```python
from build123d import *

# Parameters (mm, degrees)
SKETCH1_R           = 2.05
BOSS_EXTRUDE1_DEPTH = 4
FILLET1_R           = 1.4
CHAMFER1_SIZE       = 1.9
CUT_EXTRUDE1_DEPTH  = 1.8
SKETCH4_R           = 30
CUT_EXTRUDE2_DEPTH  = 87.446515392


with BuildPart() as part:
    # Sketch1 → Boss-Extrude1 (new body)
    with BuildSketch(Plane(origin=(0, 0, 0), x_dir=(1, 0, 0), z_dir=(0, 1, 0))):
        with BuildLine():
            Line((72.5, -41), (-72.5, -41))
            ThreePointArc((-72.5, -41), (-74.974873734, -39.974873734), (-76, -37.5))
            Line((-76, -37.5), (-76, 37.5))
            ThreePointArc((-76, 37.5), (-74.974873734, 39.974873734), (-72.5, 41))
            Line((-72.5, 41), (72.5, 41))
            ThreePointArc((72.5, 41), (74.974873734, 39.974873734), (76, 37.5))
            Line((76, 37.5), (76, -37.5))
            ThreePointArc((76, -37.5), (74.974873734, -39.974873734), (72.5, -41))
        make_face()
        with Locations(Location((-71.25, 36.2, 0), (0, 0, 270))):
            Circle(SKETCH1_R, mode=Mode.SUBTRACT)
        with Locations(Location((-71.25, -36.2, 0), (0, 0, 270))):
            Circle(SKETCH1_R, mode=Mode.SUBTRACT)
        with Locations(Location((71.25, -36.2, 0), (0, 0, 270))):
            Circle(SKETCH1_R, mode=Mode.SUBTRACT)
        with Locations(Location((71.25, 36.2, 0), (0, 0, 270))):
            Circle(SKETCH1_R, mode=Mode.SUBTRACT)
        with Locations(Location((0, 36.2, 0), (0, 0, 270))):
            Circle(SKETCH1_R, mode=Mode.SUBTRACT)
        with Locations(Location((0, -36.2, 0), (0, 0, 270))):
            Circle(SKETCH1_R, mode=Mode.SUBTRACT)
    extrude(amount=BOSS_EXTRUDE1_DEPTH)

    # Fillet1
    fillet1_edges = [part.edges().sort_by_distance(p)[0] for p in [
        (74.974873734, 4, 39.974873734),
        (76, 4, 0),
        (74.974873734, 4, -39.974873734),
        (0, 4, -41),
        (-74.974873734, 4, -39.974873734),
        (-76, 4, 0),
        (-74.974873734, 4, 39.974873734),
        (0, 4, 41),
    ]]
    fillet(fillet1_edges, radius=FILLET1_R)

    # Chamfer1
    # the kernel refuses this chamfer: 1.9 mm, written as the material it takes off along each edge
    with BuildSketch(Plane(origin=(71.25, 4, 36.2), x_dir=(0, 0, 1), z_dir=(-1, 0, 0))) as chamfer1_piece_1:
        Polygon((2.05 + CHAMFER1_SIZE, 0), (2.05, -CHAMFER1_SIZE), (2.05, 0), align=None)
    revolve(axis=Axis((71.25, 4, 36.2), (0, 1, 0)), mode=Mode.SUBTRACT)
    with BuildSketch(Plane(origin=(71.25, 4, -36.2), x_dir=(0, 0, 1), z_dir=(-1, 0, 0))) as chamfer1_piece_2:
        Polygon((2.05 + CHAMFER1_SIZE, 0), (2.05, -CHAMFER1_SIZE), (2.05, 0), align=None)
    revolve(axis=Axis((71.25, 4, -36.2), (0, 1, 0)), mode=Mode.SUBTRACT)
    with BuildSketch(Plane(origin=(-71.25, 4, 36.2), x_dir=(0, 0, 1), z_dir=(-1, 0, 0))) as chamfer1_piece_3:
        Polygon((2.05 + CHAMFER1_SIZE, 0), (2.05, -CHAMFER1_SIZE), (2.05, 0), align=None)
    revolve(axis=Axis((-71.25, 4, 36.2), (0, 1, 0)), mode=Mode.SUBTRACT)
    with BuildSketch(Plane(origin=(-71.25, 4, -36.2), x_dir=(0, 0, 1), z_dir=(-1, 0, 0))) as chamfer1_piece_4:
        Polygon((2.05 + CHAMFER1_SIZE, 0), (2.05, -CHAMFER1_SIZE), (2.05, 0), align=None)
    revolve(axis=Axis((-71.25, 4, -36.2), (0, 1, 0)), mode=Mode.SUBTRACT)
    with BuildSketch(Plane(origin=(0, 4, 36.2), x_dir=(0, 0, 1), z_dir=(-1, 0, 0))) as chamfer1_piece_5:
        Polygon((2.05 + CHAMFER1_SIZE, 0), (2.05, -CHAMFER1_SIZE), (2.05, 0), align=None)
    revolve(axis=Axis((0, 4, 36.2), (0, 1, 0)), mode=Mode.SUBTRACT)
    with BuildSketch(Plane(origin=(0, 4, -36.2), x_dir=(0, 0, 1), z_dir=(-1, 0, 0))) as chamfer1_piece_6:
        Polygon((2.05 + CHAMFER1_SIZE, 0), (2.05, -CHAMFER1_SIZE), (2.05, 0), align=None)
    revolve(axis=Axis((0, 4, -36.2), (0, 1, 0)), mode=Mode.SUBTRACT)

    # Sketch2 → Cut-Extrude1 (cut)
    with BuildSketch(Plane.XZ):
        with BuildLine():
            Line((-71.25, 33.35), (-72.5, 33.35))
            Line((-72.5, 33.35), (-72.5, -33.35))
            Line((-72.5, -33.35), (-71.25, -33.35))
            ThreePointArc((-71.25, -33.35), (-69.234745674, -34.184745674), (-68.4, -36.2))
            Line((-68.4, -36.2), (-68.4, -37.45))
            Line((-68.4, -37.45), (-2.85, -37.45))
            Line((-2.85, -37.45), (-2.85, -36.2))
            ThreePointArc((-2.85, -36.2), (0, -33.35), (2.85, -36.2))
            Line((2.85, -36.2), (2.85, -37.45))
            Line((2.85, -37.45), (68.4, -37.45))
            Line((68.4, -37.45), (68.4, -36.2))
            ThreePointArc((68.4, -36.2), (69.234745674, -34.184745674), (71.25, -33.35))
            Line((71.25, -33.35), (72.5, -33.35))
            Line((72.5, -33.35), (72.5, 33.35))
            Line((72.5, 33.35), (71.25, 33.35))
            ThreePointArc((71.25, 33.35), (69.234745674, 34.184745674), (68.4, 36.2))
            Line((68.4, 36.2), (68.4, 37.45))
            Line((68.4, 37.45), (2.85, 37.45))
            Line((2.85, 37.45), (2.85, 36.2))
            ThreePointArc((2.85, 36.2), (0, 33.35), (-2.85, 36.2))
            Line((-2.85, 36.2), (-2.85, 37.45))
            Line((-2.85, 37.45), (-68.4, 37.45))
            Line((-68.4, 37.45), (-68.4, 36.2))
            ThreePointArc((-68.4, 36.2), (-69.234745674, 34.184745674), (-71.25, 33.35))
        make_face()
    extrude(amount=-CUT_EXTRUDE1_DEPTH, mode=Mode.SUBTRACT)

    # Sketch4 → Cut-Extrude2 (cut, through all)
    with BuildSketch(Plane(origin=(0, 4, 0), x_dir=(1, 0, 0), z_dir=(0, 1, 0))):
        with Locations(Location((-35.625, 0, 0), (0, 0, 270))):
            Circle(SKETCH4_R)
        with Locations(Location((35.625, 0, 0), (0, 0, 270))):
            Circle(SKETCH4_R)
    extrude(amount=-CUT_EXTRUDE2_DEPTH, mode=Mode.SUBTRACT)


solid = part.part
```
CAD build for the part. Positions are in the model's coordinates, mm. A direction names the side the tool comes from. Round coordinates to 2 decimals unless told otherwise and drop trailing zeros. Write each loop counter-clockwise with the first axis right and the second up, starting at its lowest first coordinate (ties: lowest second). Pieces come first, ordered by that corner, then holes. Notation, with made-up numbers: (-21.5, 40.25) - (-14.5, 40.25) arc R31 cw to (-14.5, 68.25) - close; hole circle Ø1 at (-16.75, -18). An arc over 180 degrees is marked (long way). Write item = value, one per line. Start each with the question number.
Q1. Which spindle directions (+Z, -Z, +X, -X, +Y, -Y) get a long thin tool onto all of the face, cutting with end or side? Do faces 1 (the cylindrical face through (69.21, 0.89, -34.21)), 2 (the cylindrical face through (73.283, 1.035, 35.933)). Say none if no direction does.
Q2. Mould opens along X. For faces 3 (the flat face through (-1, 1, -41)), 4 (the cylindrical face through (-74.95, 1.28, 40)), 5 (the cylindrical face through (-70.634, 1.035, -34.245)) say: pulls with the +X half, pulls with the -X half, needs draft (parallel to the pull), parting line crosses it, or undercut.
Q3. Probe L1, parallel to X at y = 0.95, z = -36.2; L2, parallel to X at y = 2.4, z = 0 (3 decimals); L3, parallel to Z at x = 65, y = 1.45. List the from-to ranges inside material, lowest first. Write a range as from..to.
Q4. Band-saw the part on A-A (z = 0). Give the cut face in (x, y) (3 decimals), then the cut area to 3 significant figures.
Q5. Drop flat-ended pins along their axis: pin 1 (5.5 mm diameter, centred on x = 0, z = -36.2, fed in from +Y); pin 2 (3.5 mm diameter, centred on x = -71.25, z = -36.2, fed in from -Y); pin 3 (5.5 mm diameter, centred on x = 0, z = 36.2, fed in from -Y). Give the stop position or say it passes through.
Q6. Band-saw the part on C-C (x = 0). Give the cut face in (y, z).
Q7. Band-saw the part on D-D (z = -22). Give the cut face in (x, y).
Q8. Band-saw the part on B-B (x = 63.5). Give the cut face in (y, z), then the cut area to 3 significant figures.
Answers below:
q1.face_1 = -Y
q1.face_2 = +Y, -Y
q2.face_3 = needs draft
q2.face_4 = pulls with the -X half
q2.face_5 = undercut
q3.L1 = -76..-73.3, -69.2..-68.4, -2.85..-2.05, 2.05..2.85, 68.4..69.2, 73.3..76
q3.L2 = -76..-65.625, -5.625..5.625, 65.625..76
q3.L3 = -41..-37.45, 37.45..41
q4.outline = (-76, 0) - (-72.5, 0) - (-72.5, 1.8) - (-65.625, 1.8) - (-65.625, 4) - (-74.6, 4) arc R1.4 ccw to (-76, 2.6) - close; (-5.625, 1.8) - (5.625, 1.8) - (5.625, 4) - (-5.625, 4) - close; (65.625, 1.8) - (72.5, 1.8) - (72.5, 0) - (76, 0) - (76, 2.6) arc R1.4 ccw to (74.6, 4) - (65.625, 4) - close
q4.area = 82.2 mm2
q5.pin_1 = 2.8
q5.pin_2 = through
q5.pin_3 = 0
q6.outline = (0, -41) - (2.6, -41) arc R1.4 ccw to (3.92, -40.07) - (2.1, -38.25) - (0, -38.25) - close; (0, -34.15) - (2.1, -34.15) - (4, -32.25) - (4, 32.25) - (2.1, 34.15) - (0, 34.15) - (0, 33.35) - (1.8, 33.35) - (1.8, -33.35) - (0, -33.35) - close; (0, 38.25) - (2.1, 38.25) - (3.92, 40.07) arc R1.4 ccw to (2.6, 41) - (0, 41) - close
q7.outline = (-76, 0) - (-72.5, 0) - (-72.5, 1.8) - (-56.02, 1.8) - (-56.02, 4) - (-74.6, 4) arc R1.4 ccw to (-76, 2.6) - close; (-15.23, 1.8) - (15.23, 1.8) - (15.23, 4) - (-15.23, 4) - close; (56.02, 1.8) - (72.5, 1.8) - (72.5, 0) - (76, 0) - (76, 2.6) arc R1.4 ccw to (74.6, 4) - (56.02, 4) - close
q8.outline = (0, -41) - (2.6, -41) arc R1.4 ccw to (4, -39.6) - (4, -11.09) - (1.8, -11.09) - (1.8, -37.45) - (0, -37.45) - close; (0, 37.45) - (1.8, 37.45) - (1.8, 11.09) - (4, 11.09) - (4, 39.6) arc R1.4 ccw to (2.6, 41) - (0, 41) - close
q8.area = 144 mm2
